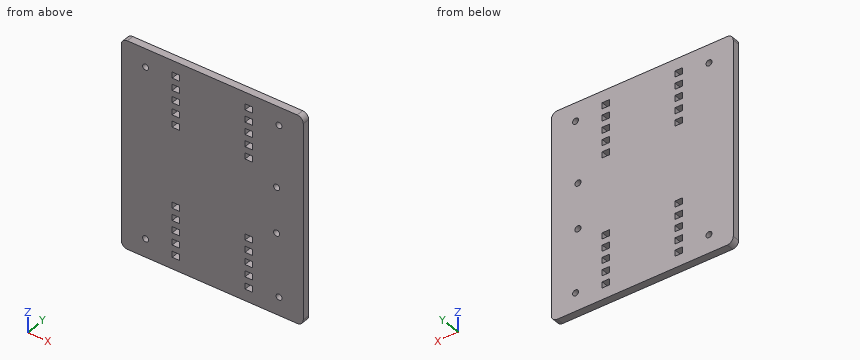
Autodesk Inventor part; units mm, degrees
ref_plane "YZ Plane" through (0, 0, 0) normal (1, 0, 0) x (0, 1, 0)
ref_plane "XZ Plane" through (0, 0, 0) normal (0, 1, 0) x (-1, 0, 0)
ref_plane "XY Plane" through (0, 0, 0) normal (0, 0, 1) x (1, 0, 0)
sketch "Sketch1" plane through (0, 0, 0) normal (0, 1, 0) x (-1, 0, 0)
  line L0 (5, 0) -> (145, 0)
  line L1 (150, -5) -> (150, -145)
  line L2 (145, -150) -> (5, -150)
  line L3 (0, -145) -> (0, -5)
  arc A0 (150, -5) -> (145, 0) centre (145, -5) ccw
  arc A1 (145, -150) -> (150, -145) centre (145, -145) ccw
  arc A2 (5, 0) -> (0, -5) centre (5, -5) ccw
  arc A3 (0, -145) -> (5, -150) centre (5, -145) ccw
  circle A4 centre (128.033, -128.033) radius 5
  circle A5 centre (128.033, -21.967) radius 5
  circle A6 centre (21.967, -21.967) radius 5
  circle A7 centre (21.967, -128.033) radius 5
  point P0 (0, 0)
  point P1 (150, -150)
  point P2 (150, 0)
  point P3 (0, -150)
  dimension "d0" = 150
  dimension "d1" = 150
  dimension "d2" = 5
  dimension "d9" = 10
  dimension "d10" = 10
  dimension "d11" = 10
  dimension "d12" = 10
extrude "Extrusion1" add sketch "Sketch1" along normal blind 6
sketch "Sketch2" plane through (0, 6, 0) normal (0, 1, 0) x (1, 0, 0)
  line L0 (0, 5) -> (0, 145)
  circle A0 centre (-21.967, 21.967) radius 5
  circle A1 centre (-21.967, 77.828) radius 11
  circle A2 centre (-37.467, 62.328) radius 1.6
  circle A3 centre (-37.467, 93.328) radius 1.6
  circle A4 centre (-6.467, 62.328) radius 1.6
  circle A5 centre (-6.467, 93.328) radius 1.6
  point P0 (0, 0)
  dimension "d15" = 22
  dimension "d21" = 3.2
  dimension "d22" = 3.2
  dimension "d23" = 3.2
  dimension "d24" = 3.2
extrude "Extrusion2" cut sketch "Sketch2" against normal blind 6 contours A1 | A2 | A3 | A4 | A5
sketch "Sketch3" plane through (0, 6, 0) normal (0, 1, 0) x (1, 0, 0)
  circle A0 centre (-128.033, 128.033) radius 5
  arc A1 (-145, 150) -> (-150, 145) centre (-145, 145) ccw
  line L0 (-150, 145) -> (0, 145)
  line L1 (0, 145) -> (0, 155)
  line L2 (-5, 160) -> (-145, 160)
  line L3 (-150, 155) -> (-150, 145)
  arc A2 (-150, 5) -> (-145, 0) centre (-145, 5) ccw
  line L4 (-150, 5) -> (0, 5)
  line L5 (0, 5) -> (0, -5)
  line L6 (-5, -10) -> (-145, -10)
  line L7 (-150, -5) -> (-150, 5)
  arc A3 (-145, 160) -> (-150, 155) centre (-145, 155) ccw
  arc A4 (0, 155) -> (-5, 160) centre (-5, 155) ccw
  arc A5 (-150, -5) -> (-145, -10) centre (-145, -5) ccw
  arc A6 (-5, -10) -> (0, -5) centre (-5, -5) ccw
  point P0 (0, 0)
  point P1 (0, 160)
  point P2 (-150, 160)
  point P3 (0, -10)
  point P4 (-150, -10)
  dimension "d29" = 150
  dimension "d30" = 15
  dimension "d31" = 150
  dimension "d32" = 15
  dimension "d33" = 5
extrude "Extrusion3" add sketch "Sketch3" against normal blind 6 contours L3 A3 L2 A4 L1 L0 | L4 L5 A6 L6 A5 L7
sketch "Sketch4" plane through (0, 6, 0) normal (0, 1, 0) x (1, 0, 0)
  circle A0 centre (-128.033, 128.033) radius 5
  line L0 (-108.033, 105.533) -> (-102.033, 105.533)
  line L1 (-102.033, 105.533) -> (-102.033, 110.533)
  line L2 (-102.033, 110.533) -> (-108.033, 110.533)
  line L3 (-108.033, 110.533) -> (-108.033, 105.533)
  circle A1 centre (-21.967, 128.033) radius 5
  line L4 (-41.967, 105.533) -> (-47.967, 105.533)
  line L5 (-47.967, 105.533) -> (-47.967, 110.533)
  line L6 (-47.967, 110.533) -> (-41.967, 110.533)
  line L7 (-41.967, 110.533) -> (-41.967, 105.533)
  circle A2 centre (-128.033, 21.967) radius 5
  line L8 (-108.033, -0.533) -> (-102.033, -0.533)
  line L9 (-102.033, -0.533) -> (-102.033, 4.467)
  line L10 (-102.033, 4.467) -> (-108.033, 4.467)
  line L11 (-108.033, 4.467) -> (-108.033, -0.533)
  circle A3 centre (-21.967, 21.967) radius 5
  line L12 (-41.967, -0.533) -> (-47.967, -0.533)
  line L13 (-47.967, -0.533) -> (-47.967, 4.467)
  line L14 (-47.967, 4.467) -> (-41.967, 4.467)
  line L15 (-41.967, 4.467) -> (-41.967, -0.533)
  point P0 (0, 0)
  dimension "d39" = 6
  dimension "d40" = 5
  dimension "d43" = 6
  dimension "d44" = 5
  dimension "d47" = 6
  dimension "d48" = 5
  dimension "d51" = 6
  dimension "d52" = 5
extrude "Extrusion4" cut sketch "Sketch4" against normal blind 6 contours L3 L2 L1 L0 | L4 L5 L6 L7 | L11 L10 L9 L8 | L12 L13 L14 L15
pattern_linear "Rectangular Pattern1" count 5 spacing 10 along (0, 0, -1) of "Extrusion4"
sketch "Sketch5" plane through (0, 6, 0) normal (0, 1, 0) x (1, 0, 0)
  circle A0 centre (-128.033, 21.967) radius 5
  circle A1 centre (-128.033, 21.967) radius 5
  circle A2 centre (-128.033, 128.033) radius 5
  circle A3 centre (-128.033, 128.033) radius 5
  circle A4 centre (-21.967, 128.033) radius 5
  circle A5 centre (-21.967, 128.033) radius 5
  circle A6 centre (-21.967, 21.967) radius 5
  circle A7 centre (-21.967, 21.967) radius 5
  point P0 (0, 0)
  dimension "d58" = 10
  dimension "d59" = 10
  dimension "d60" = 10
  dimension "d61" = 10
extrude "Extrusion5" add sketch "Sketch5" against normal blind 6
sketch "Sketch6" plane through (0, 6, 0) normal (0, 1, 0) x (1, 0, 0)
  point P0 (0, 0)
sketch "Sketch7" plane through (0, 6, 0) normal (0, 1, 0) x (1, 0, 0)
  line L0 (0, 155) -> (0, -5)
  line L1 (-44.6941, 101.1625) -> (0, 101.1625)
  line L2 (0, 101.1625) -> (0, 52.2821)
  line L3 (0, 52.2821) -> (-44.6941, 52.2821)
  line L4 (-44.6941, 52.2821) -> (-44.6941, 101.1625)
  point P0 (0, 0)
extrude "Extrusion6" add sketch "Sketch7" against normal blind 6
sketch "Sketch8" plane through (0, 6, 0) normal (0, 1, 0) x (1, 0, 0)
  line L0 (0, 155) -> (0, -5)
  circle A0 centre (-21.967, 93.65) radius 2.5
  circle A1 centre (-21.967, 56.35) radius 2.5
  point P0 (0, 0)
  dimension "d69" = 5
  dimension "d70" = 5
extrude "Extrusion7" cut sketch "Sketch8" against normal blind 6
sketch "Sketch9" plane through (0, 6, 0) normal (0, 1, 0) x (1, 0, 0)
  line L0 (-150, -5) -> (-150, 155)
  line L1 (-5, -10) -> (-145, -10)
  line L2 (-135, -10) -> (-120, -10) construction
  line L3 (0, 155) -> (0, -5)
  line L4 (0, 5) -> (15, 5) construction
  line L5 (0, 145) -> (15, 145) construction
  circle A0 centre (-130, 5) radius 2.45
  circle A1 centre (-130, 145) radius 2.45
  circle A2 centre (-20, 5) radius 2.45
  circle A3 centre (-20, 145) radius 2.45
  line L6 (-75, 75) -> (-63, 75) construction
  circle A4 centre (-83.4853, 66.5147) radius 2.75
  circle A5 centre (-83.4853, 83.4853) radius 2.75
  circle A6 centre (-66.5147, 83.4853) radius 2.75
  circle A7 centre (-66.5147, 66.5147) radius 2.75
  line L7 (-20, 5) -> (0, 5)
  line L8 (-130, 5) -> (-150, 5)
  line L9 (-130, 145) -> (-150, 145)
  line L10 (-20, 145) -> (0, 145)
  point P0 (0, 0)
  dimension "d82" = 4.9
  dimension "d83" = 4.9
  dimension "d84" = 4.9
  dimension "d85" = 4.9
  dimension "d92" = 5.5
  dimension "d93" = 5.5
  dimension "d94" = 5.5
  dimension "d95" = 5.5
  dimension "d98" = 20
  dimension "d99" = 20
  dimension "d100" = 20
  dimension "d101" = 20
extrude "Extrusion8" cut sketch "Sketch9" against normal blind 6
sketch "Sketch10" plane through (0, 6, 0) normal (0, 1, 0) x (1, 0, 0)
  line L0 (-94.8233, 59.338) -> (-53.739, 59.338)
  line L1 (-53.739, 59.338) -> (-53.739, 90.7909)
  line L2 (-53.739, 90.7909) -> (-94.8233, 90.7909)
  line L3 (-94.8233, 90.7909) -> (-94.8233, 59.338)
  point P0 (0, 0)
extrude "Extrusion9" add sketch "Sketch10" against normal blind 6
properties part number "e_bot 1"
Build history of the part. All positions in model axes, mm. Coordinates: 2 decimals unless noted, no trailing zeros. Write each loop counter-clockwise with the first axis right and the second up, starting at its lowest first coordinate (ties: lowest second). Pieces come first, ordered by that corner, then holes. Notation, with made-up numbers: (85, -24) -> (110, -24) arc R35 ccw to (110, 13) -> close; hole circle Ø4 at (29.5, -37). An arc over 180 degrees is marked (long way). Use CSV: the item, a comma, the result in double quotes. Start each with the question number.
Q1. Cut at B-B, the plane z = -42. List the corners of the cut face in (x, y).
Q2. Flat gauge pin, fed straight in: pin 1 Ø4 at (x, z) = (-21.967, -56.35) entering from -Y. Where does the tip first touch, or does it go through?
Q3. Cut at A-A, the plane x = -130. List the corners of the cut face in (y, z).
Q4. Drill centre lines: probe 1 along X at (y, z) = (0.8, -2); probe 2 along X at (y, z) = (1.4, -145); probe 3 along Z at (x, y) = (-20, 2.9). Where is each one in solid material? Low to high.
Q5. Cut at C-C, the plane y = 3.65. State how many separate pieces and enclosed holes the cut face has, then the cut area to 3 significant figures.
Checked values:
1,outline,"(-150, 0) -> (-108.03, 0) -> (-108.03, 6) -> (-150, 6) -> close; (-102.03, 0) -> (-47.97, 0) -> (-47.97, 6) -> (-102.03, 6) -> close; (-41.97, 0) -> (0, 0) -> (0, 6) -> (-41.97, 6) -> close"
2,pin 1,"passes through"
3,outline,"(0, -160) -> (6, -160) -> (6, -147.45) -> (0, -147.45) -> close; (0, -142.55) -> (6, -142.55) -> (6, -7.45) -> (0, -7.45) -> close; (0, -2.55) -> (6, -2.55) -> (6, 10) -> (0, 10) -> close"
4,probe 1,"x = -150 to -108.03, -102.03 to -47.97, -41.97 to 0"
4,probe 2,"x = -150 to -132.45, -127.55 to -22.45, -17.55 to 0"
4,probe 3,"z = -160 to -147.45, -142.55 to -95.19, -92.11 to -57.89, -54.81 to -7.45, -2.55 to 10"
5,separate pieces,"1"
5,enclosed holes,"26"
5,area,"24,800 mm²"
